Autodesk Fusion 360 part; units mm, degrees
sketch "Sketch1" plane through (0, 0, 0) normal (0, 0, 1) x (1, 0, 0)
  line L0 (0, 0) -> (28.5, 0)
  line L1 (28.5, 0) -> (28.5, 3.5)
  line L2 (28.5, 3.5) -> (0, 3.5)
  line L3 (0, 3.5) -> (0, 0)
  line L4 (-2, -2) -> (30.5, -2)
  line L5 (30.5, -2) -> (30.5, 5.5)
  line L6 (30.5, 5.5) -> (-2, 5.5)
  line L7 (-2, 5.5) -> (-2, -2)
  line L8 (-3, -8) -> (31.5, -8)
  line L9 (36.5, -3) -> (36.5, 6.5)
  line L10 (31.5, 11.5) -> (-3, 11.5)
  line L11 (-8, 6.5) -> (-8, -3)
  arc A0 (-3, 11.5) -> (-8, 6.5) centre (-3, 6.5) ccw
  arc A1 (36.5, 6.5) -> (31.5, 11.5) centre (31.5, 6.5) ccw
  arc A2 (31.5, -8) -> (36.5, -3) centre (31.5, -3) ccw
  arc A3 (-8, -3) -> (-3, -8) centre (-3, -3) ccw
  dimension "d1" = 28.5
  dimension "d2" = 3.5
  dimension "d3" = 2
  dimension "d48" = 5
extrude "Extrude1" add sketch "Sketch1" along normal blind 32.5 contours L4 L5 L6 L7
ref_plane "WorkPlane3" through (14.25, 1.75, 26) normal (0, 0, 1) x (1, 0, 0)
sketch "Sketch5" plane through (0, -2, 0) normal (0, -1, 0) x (1, 0, 0)
  line L0 (-2, 0) -> (30.5, 0)
  line L1 (30.5, 0) -> (30.5, 32.5)
  line L2 (30.5, 32.5) -> (-2, 32.5)
  line L3 (-2, 32.5) -> (-2, 0)
  line L4 (-5.25, 26) -> (33.75, 26)
  circle A0 centre (14.25, 18) radius 2.1
  line L5 (18, 21.75) -> (10.5, 21.75)
  line L6 (10.5, 21.75) -> (10.5, 14.25)
  line L7 (10.5, 14.25) -> (18, 14.25)
  line L8 (18, 14.25) -> (18, 21.75)
  line L9 (18, 21.75) -> (10.5, 14.25) construction
  line L10 (10.5, 21.75) -> (18, 14.25) construction
  line L11 (-2, 0) -> (30.5, 0)
  point P0 (14.25, 18)
  dimension "d27" = 4.2
  dimension "d28" = 7.5
  dimension "d29" = 7.5
  dimension "d30" = 8
extrude "Extrude3" add sketch "Sketch5" along normal blind 10 contours L5 L6 L7 L8
sketch "Sketch6" plane through (30.5, 0, 0) normal (1, 0, 0) x (0, 1, 0)
  line L0 (-2, 0) -> (5.5, 0)
  line L1 (5.5, 0) -> (5.5, 32.5)
  line L2 (5.5, 32.5) -> (-2, 32.5)
  line L3 (-2, 32.5) -> (-2, 0)
  line L4 (6.25, 26) -> (-2.75, 26)
  circle A0 centre (1.75, 30) radius 1.25
  line L5 (1.75, 31.25) -> (1.75, 28.75)
  dimension "d36" = 2.5
  dimension "d37" = 3.75
  dimension "d38" = 2.5
  dimension "d39" = 2.5
revolve "Revolve1" cut sketch "Sketch6" angle 360 about axis through (30.5, 1.75, 31.25) along (0, 0, -1) contours A0 L5 picked at (2.4551, 29.6422)
sketch "Sketch7" plane through (-2, 0, 0) normal (-1, 0, 0) x (0, -1, 0)
  line L0 (-5.5, 0) -> (2, 0)
  line L1 (2, 0) -> (2, 32.5)
  line L2 (2, 32.5) -> (-5.5, 32.5)
  line L3 (-5.5, 32.5) -> (-5.5, 0)
  line L4 (-6.25, 26) -> (2.75, 26)
  circle A0 centre (-1.75, 30) radius 1.25
  line L5 (-1.75, 31.25) -> (-1.75, 28.75)
  point P0 (-1.75, 31.25)
  dimension "d41" = 2.5
  dimension "d42" = 3.75
  dimension "d43" = 2.5
revolve "Revolve2" cut sketch "Sketch7" angle 360 about axis through (-2, 1.75, 31.25) along (0, 0, -1) contours A0 L5 picked at (-1.2448, 29.6517)
extrude "Extrude4" add sketch "Sketch1" along normal blind 0.25 contours L8 L9 L10 L11 A0 A1 A2 A3
sketch "Sketch8" plane through (14.25, 1.75, 26) normal (0, 0, 1) x (1, 0, 0)
  line L0 (16.25, -3.75) -> (16.25, 3.75)
  line L1 (16.25, -3.75) -> (30.25, -3.75)
  line L2 (30.25, -3.75) -> (30.25, 3.75)
  line L3 (30.25, 3.75) -> (16.25, 3.75)
  line L4 (16.25, 3.75) -> (16.25, -3.75)
  circle A0 centre (26.5, 0) radius 2.05
  circle A1 centre (26.5, 0) radius 3.55
  line L5 (-14.25, -1.75) -> (14.25, -1.75)
  line L6 (14.25, 1.75) -> (-14.25, 1.75)
  line L7 (0, -1.75) -> (0, 1.75)
  line L8 (-16.25, -3.75) -> (-16.25, 3.75)
  line L9 (-16.25, 3.75) -> (-16.25, -3.75)
  line L10 (-16.25, -3.75) -> (-30.25, -3.75)
  line L11 (-30.25, -3.75) -> (-30.25, 3.75)
  circle A2 centre (-26.5, 0) radius 2.05
  line L12 (-30.25, 3.75) -> (-16.25, 3.75)
  circle A3 centre (-26.5, 0) radius 3.55
  dimension "d51" = 7.5
  dimension "d52" = 14
  dimension "d53" = 4.1
  dimension "d54" = 3.75
  dimension "d55" = 3.75
  dimension "d56" = 7.1
extrude "Extrude6" add sketch "Sketch8" against normal blind 3 contours L0 L1 L2 L3 L4 | A0 | A1 | L8 L9 L10 L11 L12 | A2 | A3
chamfer "Chamfer3" distance 10 distance2 10 1 edges at (14.25, -2, 14.25) measured on face at (13, -2, 4.9167)
chamfer "Chamfer4" distance 14 angle 45 2 edges at (-2, 1.75, 23) (30.5, 1.75, 23)
extrude "Extrude7" cut sketch "Sketch8" against normal blind 4 contours A0 | A2
equation "d6 = 26 mm + 1.5 mm + 5 mm"
equation "d39 = d36"
equation "d54 = d51 / 2"
equation "d55 = d54"
equation "d56 = d53 + 3 mm"
Here's how the part is built. I have some questions about the finished solid (model axes, mm). A direction names the side the tool comes from. Round coordinates to 2 decimals unless told otherwise and drop trailing zeros. Loops run counter-clockwise (first coordinate to the right, second up) from the corner with the lowest first, then second, coordinate; pieces in that order, holes last. Notation, with made-up numbers: (-22.5, -11.5) - (-10.5, -11.5) arc R21 cw to (-10.5, 0.5) - close; hole circle Ø7 at (59, 46.25). An arc over 180 degrees is marked (long way). One line per question, with ' | ' between items. Start each with the question number.
Q1. Will these pins go through, and if not, where does the flat tip stop? pin 1 (12 mm diameter, centred on y = 0, z = 4.5, fed in from -X); pin 2 (3.5 mm diameter, centred on x = 41, y = 2.5, fed in from +Z); pin 3 (2 mm diameter, centred on y = 2, z = 29.5, fed in from +X).
Q2. Please list where these lines run through material, in increasing order: line 1 (Y direction, x = 2, z = 2); line 2 (Y direction, x = 13, z = 21.5); line 3 (Y direction, x = -7.5, z = 16.5). Write a range as [from, to].
Q3. We'd pull the mould along Z, two halves only. Please class faces 1 (the flat face through (30.5, 2, 5)), 2 (the cylindrical face through (13.977, -6.93, 15.918)), 3 (the flat face through (13.9, -0.3, 0)), 4 (the flat face through (-12, 2, 22)): +Z half, -Z half, draft (parallel to the pull), parting line (faces both ways), or undercut.
Q4. For faces 5 (the flat face through (-9, 2, 26)), 6 (the flat face through (30.5, 2, 28)), 7 (the flat face through (14, 3.5, 16)), 8 (the cylindrical face through (-14.3, 1.8, 24)), 9 (the flat face through (-9, 2, 16)), which set-ups out of +Z, -Z, +X, -X, +Y, -Y let a thin tool reach every point of the face, with its end or its side?
Q5. I want a section at D-D (y = -4.25). Write out the boundary of the cut face in (x, z).
Q6. I want a section at C-C (z = 25). Write out the boundary of the cut face in (x, y), then the cut area to 3 significant figures.
Response values:
1) pin 1: stops at x = -8 | pin 2: stops at z = 26 | pin 3: stops at x = 30.5
2) line 1: y = [-2, 0], [3.5, 5.5] | line 2: y = [-12, 0], [3.5, 5.5] | line 3: y = [-2, 5.5]
3) face 1: undercut | face 2: undercut | face 3: -Z half | face 4: +Z half
4) face 5: +Z, -X, +Y, -Y | face 6: +Z, +X, +Y, -Y | face 7: +Z, -Z | face 8: +Z | face 9: -X, +Y, -Y
5) outline: (-7.84, 0) - (36.34, 0) - (36.34, 0.25) - (-7.84, 0.25) - close; (10.5, 6.5) - (18, 6.5) - (18, 21.75) - (10.5, 21.75) - close; hole circle Ø4.2 at (14.25, 18)
6) outline: (-16, -2) - (44.5, -2) - (44.5, 5.5) - (-16, 5.5) - close; hole circle Ø4.1 at (-12.25, 1.75); hole (0, 0) - (28.5, 0) - (28.5, 3.5) - (0, 3.5) - close; hole circle Ø4.1 at (40.75, 1.75) | area: 328 mm²
